Build history of the part. All positions in model axes, mm. A direction names the side the tool comes from. Round coordinates to 2 decimals unless told otherwise and drop trailing zeros. Write each loop counter-clockwise with the first axis right and the second up, starting at its lowest first coordinate (ties: lowest second). Pieces come first, ordered by that corner, then holes.
1) Saw through at C-C (y = 105). Write the cut outline in (x, z).
2) Flat gauge pins, fed straight in: pin 1 (6 mm diameter, centred on x = -55, z = 10.5, fed in from +Y); pin 2 (6 mm diameter, centred on y = 88.5, z = 2.5, fed in from -X); pin 3 (2 mm diameter, centred on x = -158.5, z = 7.5, fed in from +Y). Where does each tip first touch, or does it go through?
3) Wall check: probe 1 along Y at (x, z) = (-142, 11); probe 2 along Y at (x, z) = (7, 10); probe 3 along Y at (x, z) = (-58.5, 9.5). Give the ranges that are in metal, low to high.
4) Pull direction Y, two halves, no side cores. Call faces 1 (the flat face through (-37.347, 84.685, 6.261)), 2 (the flat face through (-178.962, 79.254, 6.261)), 3 (the flat face through (13.472, 83.273, 6.261)), 4 (the flat face through (-83, 79, 0)): +Y half, -Y half, draft (parallel to the pull), parting line (faces both ways), or undercut.
5) Which spindle directions (+Z, -Z, +X, -X, +Y, -Y) get a long thin tool onto all of the face, cutting with end or side? Do faces 5 (the cylindrical face through (-43.88, 80.26, 6.26)), 6 (the flat face through (-191, 66.762, 6)). Say none if no direction does.
6) Saw through at A-A (z = 4.25). State how many separate pieces and enclosed holes the cut face has, plus the area to 3 significant figures.
7) Saw through at B-B (x = -164). Write the cut outline in (y, z), plus the area to 3 significant figures.
from build123d import *

# Parameters (mm, degrees)
SKETCH1_R           = 3.2639
SKETCH1_R_2         = 4.8025
BOSS_EXTRUDE1_DEPTH = 12.7
SKETCH2_R           = 1.5
CUT_EXTRUDE1_DEPTH  = 227.41953776
EXTRUDE_THIN1_DEPTH = 12.7
FILLET1_R           = 2
FILLET2_R           = 1
FILLET3_R           = 1
FILLET4_R           = 2
FILLET5_R           = 1


with BuildPart() as part:
    # Sketch1 → Boss-Extrude1 (new body)
    with BuildSketch(Plane.XY):
        with BuildLine():
            Line((-196.801436578, 66.762186411), (-184.101436578, 66.762186411))
            Line((-184.101436578, 66.762186411), (-174.101436578, 68.762186411))
            Line((-174.101436578, 68.762186411), (18.198563422, 71.262186411))
            Line((18.198563422, 71.262186411), (29.067448443, 79.140508783))
            ThreePointArc((29.067448443, 79.140508783), (32.782860984, 90.090472281), (23.683493494, 97.225421632))
            Line((23.683493494, 97.225421632), (22.457622919, 111.237186411))
            Line((22.457622919, 111.237186411), (12.506829792, 94.001907138))
            Line((12.506829792, 94.001907138), (-157.097736409, 82.762186411))
            Line((-157.097736409, 82.762186411), (-153.097736409, 91.762186411))
            Line((-153.097736409, 91.762186411), (-161.097736409, 91.762186411))
            Line((-161.097736409, 91.762186411), (-196.801436578, 66.762186411))
        make_face()
        with Locations((-141.801436578, 76.478988882)):
            Circle(SKETCH1_R, mode=Mode.SUBTRACT)
        with BuildLine():
            ThreePointArc((-121.040083953, 77.299723999), (-124.172509206, 73.909444003), (-127.562789202, 77.041869256))
            ThreePointArc((-127.562789202, 77.041869256), (-124.430363949, 80.432149252), (-121.040083953, 77.299723999))
        make_face(mode=Mode.SUBTRACT)
        with BuildLine():
            ThreePointArc((-103.540083953, 77.991531744), (-106.672509206, 74.601251748), (-110.062789202, 77.733677001))
            ThreePointArc((-110.062789202, 77.733677001), (-106.930363949, 81.123956997), (-103.540083953, 77.991531744))
        make_face(mode=Mode.SUBTRACT)
        with BuildLine():
            ThreePointArc((-86.040083953, 78.68333949), (-89.172509206, 75.293059493), (-92.562789202, 78.425484746))
            ThreePointArc((-92.562789202, 78.425484746), (-89.430363949, 81.815764743), (-86.040083953, 78.68333949))
        make_face(mode=Mode.SUBTRACT)
        with BuildLine():
            ThreePointArc((-68.540083953, 79.375147235), (-71.672509206, 75.984867239), (-75.062789202, 79.117292491))
            ThreePointArc((-75.062789202, 79.117292491), (-71.930363949, 82.507572488), (-68.540083953, 79.375147235))
        make_face(mode=Mode.SUBTRACT)
        with Locations((-54.301436578, 79.938027609)):
            Circle(SKETCH1_R, mode=Mode.SUBTRACT)
        with BuildLine():
            ThreePointArc((-39.833809225, 76.508242407), (-43.882673124, 80.349599411), (-40.150307356, 84.499149782))
            Line((-40.150307356, 84.499149782), (11.706060944, 87.935679297))
            Line((11.706060944, 87.935679297), (15.760597764, 77.230998609))
            Line((15.760597764, 77.230998609), (-39.833809225, 76.508242407))
        make_face(mode=Mode.SUBTRACT)
        with Locations((23.198563422, 87.237186411)):
            Circle(SKETCH1_R_2, mode=Mode.SUBTRACT)
    extrude(amount=BOSS_EXTRUDE1_DEPTH)

    # Sketch2 → Cut-Extrude1 (cut, through all)
    with BuildSketch(Plane.XY.offset(12.7)):
        with Locations((11.978454756, 94.850918223)):
            Circle(SKETCH2_R)
    extrude(amount=-CUT_EXTRUDE1_DEPTH, mode=Mode.SUBTRACT)

    # Sketch3 → Extrude-Thin1 (add)
    with BuildSketch(Plane.XY.offset(12.7)):
        Polygon((4.374887162, 91.481339263), (2.874887162, 88.883263052), (-3.183006438, 78.390683549), (-4.683006438, 75.792607338), (0.080133283, 73.042607338), (1.580133283, 75.640683549), (7.638026883, 86.133263052), (9.138026883, 88.731339263), align=None)
        Polygon((-6.366359526, 74.910825854), (-8.455450886, 78.321939644), (-14.081085771, 87.507598585), (-16.170177131, 90.918712375), (-20.860458592, 88.046211754), (-18.771367232, 84.635097964), (-13.145732348, 75.449439024), (-11.056640987, 72.038325234), align=None)
        Polygon((-28.307796362, 89.315452792), (-29.807796362, 86.71737658), (-34.852924598, 77.978958144), (-36.352924598, 75.380881933), (-31.589784877, 72.630881933), (-30.089784877, 75.228958144), (-25.044656641, 83.96737658), (-23.544656641, 86.565452792), align=None)
    extrude(amount=-EXTRUDE_THIN1_DEPTH)

    # Fillet1
    fillet1_edges = [part.edges().sort_by_distance(p)[0] for p in [
        (-4.000877594, 76.974089152, 6.35),
        (1.954701783, 87.289455223, 6.35),
        (2.398004439, 77.057277946, 6.35),
        (8.558212262, 87.72707088, 6.35),
        (-13.999872127, 76.844097024, 6.35),
        (-19.525203724, 85.865978577, 6.35),
        (-7.601311108, 76.927281645, 6.35),
        (-13.327249279, 86.276717973, 6.35),
        (-35.670795755, 76.562363747, 6.35),
        (-30.727981741, 85.123568752, 6.35),
        (-29.271913721, 76.645552541, 6.35),
        (-24.124471262, 85.561184409, 6.35),
        (15.760597764, 77.230998609, 6.35),
        (11.706060944, 87.935679297, 6.35),
    ]]
    fillet(fillet1_edges, radius=FILLET1_R)

    # Fillet2
    fillet2_edges = [part.edges().sort_by_distance(p)[0] for p in [
        (13.348980962, 95.460555753, 6.35),
        (10.826213816, 93.890532459, 6.35),
    ]]
    fillet(fillet2_edges, radius=FILLET2_R)

    # Fillet3
    fillet3_edges = [part.edges().sort_by_distance(p)[0] for p in [
        (-157.097736409, 82.762186411, 6.35),
    ]]
    fillet(fillet3_edges, radius=FILLET3_R)

    # Fillet4
    fillet4_edges = [part.edges().sort_by_distance(p)[0] for p in [
        (-161.097736409, 91.762186411, 6.35),
    ]]
    fillet(fillet4_edges, radius=FILLET4_R)

    # Fillet5
    fillet5_edges = [part.edges().sort_by_distance(p)[0] for p in [
        (22.457622919, 111.237186411, 6.35),
        (23.683493494, 97.225421632, 6.35),
    ]]
    fillet(fillet5_edges, radius=FILLET5_R)


solid = part.part
Evaluation:
1. outline: (18.86, 0) - (23, 0) - (23, 12.7) - (18.86, 12.7) - close
2. pin 1: stops at y = 89.73
2. pin 2: stops at x = -170.04
2. pin 3: stops at y = 91.76
3. probe 1: y = 69.18 to 73.22, 79.74 to 83.76
3. probe 2: y = 71.12 to 77.12, 85.03 to 93.64
3. probe 3: y = 70.27 to 89.3
4. face 1: undercut
4. face 2: +Y half
4. face 3: undercut
4. face 4: draft
5. face 5: +Z, -Z
5. face 6: +Z, -Z, +X, -X, -Y
6. separate pieces: 1
6. enclosed holes: 11
6. area: 3,510 mm2
7. outline: (68.89, 0) - (89.73, 0) - (89.73, 12.7) - (68.89, 12.7) - close
7. area: 265 mm2
